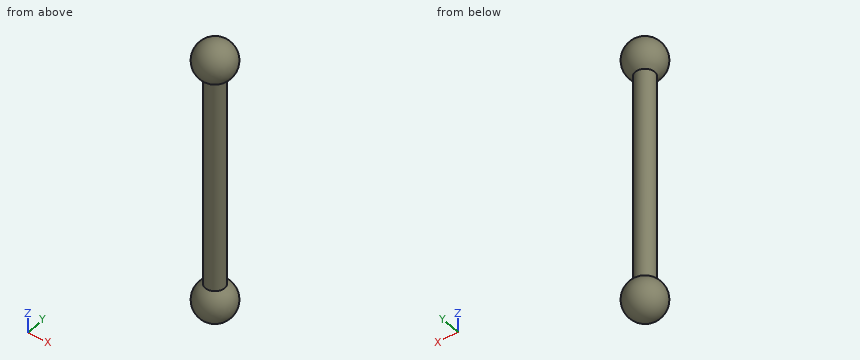
from build123d import *

# Parameters (mm, degrees)
SKETCH1_R           = 2
BOSS_EXTRUDE1_DEPTH = 45


with BuildPart() as part:
    # Sketch1 → Boss-Extrude1 (new body)
    with BuildSketch(Plane.XY):
        Circle(SKETCH1_R)
    extrude(amount=-BOSS_EXTRUDE1_DEPTH)

    # Sketch2 → Revolve1 (revolve)
    with BuildSketch(Plane.XY.offset(3)):
        with BuildLine():
            Line((0, 4), (0, -4))
            ThreePointArc((0, -4), (4, 0), (0, 4))
        make_face()
    revolve1 = revolve(axis=Axis((0, 4, 3), (0, -1, 0)))

    # Mirror2: Revolve1 across plane
    add(revolve1.mirror(Plane.XY.offset(-22.5)))


solid = part.part
Verification items for the finished model (mm, model axes). Give positions to 0.01 mm unless a question says otherwise; leave off trailing zeros. Write each loop counter-clockwise with the first axis right and the second up, starting at its lowest first coordinate (ties: lowest second). Pieces come first, ordered by that corner, then holes. Notation, with made-up numbers: (7.5, 42.25) -> (16.5, 42.25) arc R21 cw to (16.5, 53.25) -> close; hole circle Ø10 at (40, 0). An arc over 180 degrees is marked (long way). Use CSV: the item, a comma, the result in double quotes.
(1) Sectioned sample at A-A (x = 3.25). Record the cut outline in (y, z).
Derived:
outline,"circle Ø4.66 at (0, -48); circle Ø4.66 at (0, 3)"
(2) Material ranges on L1, parallel to Z at x = 0.5, y = 2.75; L2, parallel to Z at x = -3.5, y = 0.75; L3, parallel to X at y = 1.75, z = -0.5, recorded low to high.
Derived:
L1,"z = -50.86 to -45.14, 0.14 to 5.86"
L2,"z = -49.79 to -46.21, 1.21 to 4.79"
L3,"x = -0.97 to 0.97"
(3) Sectioned sample at D-D (x = 0). Record the cut outline in (y, z).
Derived:
outline,"(-2, -44.54) arc R4 ccw (long way) to (2, -44.54) -> (2, -0.46) arc R4 ccw (long way) to (-2, -0.46) -> close"
(4) Go/stop test with flat-tipped pins: pin 1 (2 mm diameter, centred on x = 2, y = 0.5, fed in from +Z); pin 2 (1.5 mm diameter, centred on y = -0.5, z = -8.5, fed in from -X); pin 3 (2 mm diameter, centred on x = -0.5, y = 1.5, fed in from +Z). Record where each tip stops, or that it passes through.
Derived:
pin 1,"stops at z = 6.86"
pin 2,"stops at x = -2"
pin 3,"stops at z = 6.96"
(5) Sectioned sample at C-C (z = -42.5). Record the cut outline in (x, y).
Derived:
outline,"circle Ø4 at (0, 0)"
(6) Sectioned sample at B-B (y = 3.5). Record the cut outline in (x, z), plus the area to 3 significant figures.
Derived:
outline,"circle Ø3.87 at (0, -48); circle Ø3.87 at (0, 3)"
area,"23.6 mm^2"
